Model file for the job. Use its own axes, mm. A direction names the side the tool comes from. Round coordinates to 2 decimals unless told otherwise and drop trailing zeros. Loops run counter-clockwise (first coordinate to the right, second up) from the corner with the lowest first, then second, coordinate; pieces in that order, holes last. Notation, with made-up numbers: (6, 0) - (42, 0) arc R33 cw to (42, 29) - close; hole circle Ø4 at (73, -22.5). An arc over 180 degrees is marked (long way). Answer as a JSON object with one key per item and string values.
from build123d import *

# Parameters (mm, degrees)
BOSS_EXTRUDE1_DEPTH     = 5
SKETCH4_W               = 80
SKETCH4_H               = 80
BOSS_EXTRUDE2_DEPTH     = 5
CUT_EXTRUDE4_DEPTH      = 5
CUT_EXTRUDE4_DEPTH_BACK = 5
SKETCH6_R               = 2.5
SKETCH7_R               = 1.25
CUT_EXTRUDE5_DEPTH      = 5
SKETCH8_R               = 5
CUT_EXTRUDE6_DEPTH      = 10
BOSS_EXTRUDE3_START     = -5
BOSS_EXTRUDE3_DEPTH     = 5
FILLET1_R               = 2
FILLET2_R               = 2


with BuildPart() as part:
    # Sketch3 → Boss-Extrude1 (new body)
    with BuildSketch(Plane(origin=(0, 0, 0), x_dir=(1, 0, 0), z_dir=(0, 1, 0))):
        with BuildLine():
            Line((-60, 40), (-40, 60))
            ThreePointArc((-40, 60), (0, 42.5), (40, 60))
            Line((40, 60), (60, 40))
            ThreePointArc((60, 40), (42.5, 0), (60, -40))
            Line((60, -40), (40, -60))
            ThreePointArc((40, -60), (0, -42.5), (-40, -60))
            Line((-40, -60), (-60, -40))
            ThreePointArc((-60, -40), (-42.5, 0), (-60, 40))
        make_face()
    extrude(amount=BOSS_EXTRUDE1_DEPTH)

    # Sketch4 → Boss-Extrude2 (add)
    with BuildSketch(Plane(origin=(0, 5, 0), x_dir=(1, 0, 0), z_dir=(0, 1, 0))):
        Rectangle(SKETCH4_W, SKETCH4_H)
    extrude(amount=BOSS_EXTRUDE2_DEPTH)

    # Sketch6 → Cut-Extrude4 (cut, two sides: drawn at the far end of the back side and taken through both)
    with BuildSketch(Plane(origin=(0, 5, 0), x_dir=(1, 0, 0), z_dir=(0, 1, 0)).offset(-CUT_EXTRUDE4_DEPTH_BACK)):
        with Locations(Location((-35, 35, 0), (0, 0, 270))):
            Circle(SKETCH6_R)
        with Locations(Location((35, 35, 0), (0, 0, 90))):
            Circle(SKETCH6_R)
        with Locations(Location((35, -35, 0), (0, 0, 270))):
            Circle(SKETCH6_R)
        with Locations(Location((-35, -35, 0), (0, 0, 90))):
            Circle(SKETCH6_R)
    extrude(amount=CUT_EXTRUDE4_DEPTH + CUT_EXTRUDE4_DEPTH_BACK, mode=Mode.SUBTRACT)

    # Sketch7 → Cut-Extrude5 (cut)
    with BuildSketch(Plane(origin=(0, 5, 0), x_dir=(1, 0, 0), z_dir=(0, 1, 0))):
        with BuildLine():
            Line((-47.878679656, 50.707106781), (-49.292893219, 49.292893219))
            Line((-49.292893219, 49.292893219), (-40.807611845, 40.807611845))
            Line((-40.807611845, 40.807611845), (-39.393398282, 42.221825407))
            ThreePointArc((-39.393398282, 42.221825407), (-39.100505063, 42.928932188), (-39.393398282, 43.636038969))
            Line((-39.393398282, 43.636038969), (-46.464466094, 50.707106781))
            ThreePointArc((-46.464466094, 50.707106781), (-47.171572875, 51), (-47.878679656, 50.707106781))
        make_face()
        with BuildLine():
            Line((-40.807611845, 40.807611845), (-49.292893219, 49.292893219))
            Line((-49.292893219, 49.292893219), (-50.707106781, 47.878679656))
            ThreePointArc((-50.707106781, 47.878679656), (-51, 47.171572875), (-50.707106781, 46.464466094))
            Line((-50.707106781, 46.464466094), (-43.636038969, 39.393398282))
            ThreePointArc((-43.636038969, 39.393398282), (-42.928932188, 39.100505063), (-42.221825407, 39.393398282))
            Line((-42.221825407, 39.393398282), (-40.807611845, 40.807611845))
        make_face()
        with Locations(Location((-53.181980515, 41.868272016, 0), (0, 0, 270))):
            Circle(SKETCH7_R)
        with Locations(Location((-48.232233047, 36.918524548, 0), (0, 0, 270))):
            Circle(SKETCH7_R)
        with Locations(Location((-41.868272016, 53.181980515, 0), (0, 0, 270))):
            Circle(SKETCH7_R)
        with Locations(Location((-36.918524548, 48.232233047, 0), (0, 0, 270))):
            Circle(SKETCH7_R)
        with BuildLine():
            Line((-39.393398282, -42.221825407), (-40.807611845, -40.807611845))
            Line((-40.807611845, -40.807611845), (-49.292893219, -49.292893219))
            Line((-49.292893219, -49.292893219), (-47.878679656, -50.707106781))
            ThreePointArc((-47.878679656, -50.707106781), (-47.171572875, -51), (-46.464466094, -50.707106781))
            Line((-46.464466094, -50.707106781), (-39.393398282, -43.636038969))
            ThreePointArc((-39.393398282, -43.636038969), (-39.100505063, -42.928932188), (-39.393398282, -42.221825407))
        make_face()
        with BuildLine():
            Line((-49.292893219, -49.292893219), (-40.807611845, -40.807611845))
            Line((-40.807611845, -40.807611845), (-42.221825407, -39.393398282))
            ThreePointArc((-42.221825407, -39.393398282), (-42.928932188, -39.100505063), (-43.636038969, -39.393398282))
            Line((-43.636038969, -39.393398282), (-50.707106781, -46.464466094))
            ThreePointArc((-50.707106781, -46.464466094), (-51, -47.171572875), (-50.707106781, -47.878679656))
            Line((-50.707106781, -47.878679656), (-49.292893219, -49.292893219))
        make_face()
        with Locations(Location((-53.181980515, -41.868272016, 0), (0, 0, 270))):
            Circle(SKETCH7_R)
        with Locations(Location((-48.232233047, -36.918524548, 0), (0, 0, 270))):
            Circle(SKETCH7_R)
        with Locations(Location((-41.868272016, -53.181980515, 0), (0, 0, 270))):
            Circle(SKETCH7_R)
        with BuildLine():
            Line((49.292893219, -49.292893219), (40.807611845, -40.807611845))
            Line((40.807611845, -40.807611845), (39.393398282, -42.221825407))
            ThreePointArc((39.393398282, -42.221825407), (39.100505063, -42.928932188), (39.393398282, -43.636038969))
            Line((39.393398282, -43.636038969), (46.464466094, -50.707106781))
            ThreePointArc((46.464466094, -50.707106781), (47.171572875, -51), (47.878679656, -50.707106781))
            Line((47.878679656, -50.707106781), (49.292893219, -49.292893219))
        make_face()
        with BuildLine():
            Line((42.221825407, -39.393398282), (40.807611845, -40.807611845))
            Line((40.807611845, -40.807611845), (49.292893219, -49.292893219))
            Line((49.292893219, -49.292893219), (50.707106781, -47.878679656))
            ThreePointArc((50.707106781, -47.878679656), (51, -47.171572875), (50.707106781, -46.464466094))
            Line((50.707106781, -46.464466094), (43.636038969, -39.393398282))
            ThreePointArc((43.636038969, -39.393398282), (42.928932188, -39.100505063), (42.221825407, -39.393398282))
        make_face()
        with Locations(Location((53.181980515, -41.868272016, 0), (0, 0, 270))):
            Circle(SKETCH7_R)
        with BuildLine():
            Line((39.393398282, 42.221825407), (40.807611845, 40.807611845))
            Line((40.807611845, 40.807611845), (49.292893219, 49.292893219))
            Line((49.292893219, 49.292893219), (47.878679656, 50.707106781))
            ThreePointArc((47.878679656, 50.707106781), (47.171572875, 51), (46.464466094, 50.707106781))
            Line((46.464466094, 50.707106781), (39.393398282, 43.636038969))
            ThreePointArc((39.393398282, 43.636038969), (39.100505063, 42.928932188), (39.393398282, 42.221825407))
        make_face()
        with BuildLine():
            Line((49.292893219, 49.292893219), (40.807611845, 40.807611845))
            Line((40.807611845, 40.807611845), (42.221825407, 39.393398282))
            ThreePointArc((42.221825407, 39.393398282), (42.928932188, 39.100505063), (43.636038969, 39.393398282))
            Line((43.636038969, 39.393398282), (50.707106781, 46.464466094))
            ThreePointArc((50.707106781, 46.464466094), (51, 47.171572875), (50.707106781, 47.878679656))
            Line((50.707106781, 47.878679656), (49.292893219, 49.292893219))
        make_face()
        with Locations(Location((41.868272016, 53.181980515, 0), (0, 0, 270))):
            Circle(SKETCH7_R)
        with Locations(Location((36.918524548, 48.232233047, 0), (0, 0, 270))):
            Circle(SKETCH7_R)
        with Locations(Location((53.181980515, 41.868272016, 0), (0, 0, 270))):
            Circle(SKETCH7_R)
        with Locations(Location((48.232233047, 36.918524548, 0), (0, 0, 270))):
            Circle(SKETCH7_R)
        with Locations(Location((-36.918524548, -48.232233047, 0), (0, 0, 90))):
            Circle(SKETCH7_R)
        with Locations(Location((48.232233047, -36.918524548, 0), (0, 0, 90))):
            Circle(SKETCH7_R)
        with Locations(Location((41.868272016, -53.181980515, 0), (0, 0, 270))):
            Circle(SKETCH7_R)
        with Locations(Location((36.918524548, -48.232233047, 0), (0, 0, 270))):
            Circle(SKETCH7_R)
    extrude(amount=-CUT_EXTRUDE5_DEPTH, mode=Mode.SUBTRACT)

    # Sketch8 → Cut-Extrude6 (cut)
    with BuildSketch(Plane(origin=(0, 0, 0), x_dir=(1, 0, 0), z_dir=(0, 1, 0))):
        with Locations(Location((0, 0, 0), (0, 0, 270))):
            Circle(SKETCH8_R)
    extrude(amount=CUT_EXTRUDE6_DEPTH, mode=Mode.SUBTRACT)

    # Sketch9 → Boss-Extrude3 (add)
    with BuildSketch(Plane(origin=(0, 5, 0), x_dir=(1, 0, 0), z_dir=(0, 1, 0)).offset(BOSS_EXTRUDE3_START)):
        with BuildLine():
            Line((-15, -96.964285714), (15, -96.964285714))
            add(Edge.make_bspline(
                [(15, -96.964285714), (15.040974101, -60.242963076), (40, -60)],
                knots=[0, 0, 0, 1, 1, 1], degree=2))
            ThreePointArc((40, -60), (0, -42.5), (-40, -60))
            add(Edge.make_bspline(
                [(-15, -96.964285714), (-15.040974101, -60.242963076), (-40, -60)],
                knots=[0, 0, 0, 1, 1, 1], degree=2))
        make_face()
    extrude(amount=BOSS_EXTRUDE3_DEPTH)

    # Fillet1
    fillet1_edges = [part.edges().sort_by_distance(p)[0] for p in [
        (-40, 2.5, 60),
        (-60, 2.5, 40),
        (-60, 2.5, -40),
        (-40, 2.5, -60),
        (40, 2.5, -60),
        (60, 2.5, -40),
        (-15, 2.5, 96.964285714),
        (60, 2.5, 40),
        (40, 2.5, 60),
        (15, 2.5, 96.964285714),
    ]]
    fillet(fillet1_edges, radius=FILLET1_R)

    # Fillet2
    fillet2_edges = [part.edges().sort_by_distance(p)[0] for p in [
        (40, 7.5, 40),
        (40, 7.5, -40),
        (-40, 7.5, -40),
        (-40, 7.5, 40),
    ]]
    fillet(fillet2_edges, radius=FILLET2_R)


solid = part.part
1) Probe probe 1 along Y at (x, z) = (-9, 89); probe 2 along Z at (x, y) = (-28, 8.75); probe 3 along X at (y, z) = (2, 8). List the from-to ranges inside material, lowest first.
Values follow:
{"probe 1": "0 to 5", "probe 2": "-40 to 40", "probe 3": "-43.09 to 43.09"}
2) Tool access for faces 4 (the flat face through (42.88, 2.54, 47.12)), 5 (the flat face through (-1, 7, 40)), 6 (the flat face through (-1, 7, -40)): list every direction of +Z, -Z, +X, -X, +Y, -Y with a clear straight run to the whole face (end or side of a thin tool).
Values follow:
{"face 4": "+Y, -Y", "face 5": "+Z, +X, -X, +Y", "face 6": "-Z, +X, -X, +Y"}
3) Slice it at A-A on z = 0. List the corners of the cut face in (x, y), then the cut area to 3 significant figures.
Values follow:
{"outline": "(-42.5, 0) - (-5, 0) - (-5, 10) - (-40, 10) - (-40, 5) - (-42.5, 5) - close; (5, 0) - (42.5, 0) - (42.5, 5) - (40, 5) - (40, 10) - (5, 10) - close", "area": "725 mm²"}
4) Slice it at B-B on y = 7. List the corners of the cut face in (x, z), then the cut area to 3 significant figures.
Values follow:
{"outline": "(-40, -38) arc R2 ccw to (-38, -40) - (38, -40) arc R2 ccw to (40, -38) - (40, 38) arc R2 ccw to (38, 40) - (-38, 40) arc R2 ccw to (-40, 38) - close; hole circle Ø5 at (-35, -35); hole circle Ø5 at (-35, 35); hole circle Ø10 at (0, 0); hole circle Ø5 at (35, -35); hole circle Ø5 at (35, 35)", "area": "6,240 mm²"}
5) Drop flat-ended pins along their axis: P1, Ø1.5, axis at x = -36.92, z = 48.23, coming from the +Y side; P2, Ø5, axis at y = 5, z = -8, coming from the +X side; P3, Ø2, axis at x = -24, y = 5.5, coming from the +Z side; P4, Ø2, axis at y = 2, z = 23.5, coming from the +X side. Give the stop position or say it passes through.
Values follow:
{"P1": "through", "P2": "x = 43.52", "P3": "z = 66.96", "P4": "x = 48.32"}
6) Two-plate mould, pull along X, no slides. Class faces 1 (the flat face through (-40, 7, 1)), 2 (the flat face through (40, 7, 1)), 3 (the cylindrical face through (34.249, 4.93, -37.385)): pulls with the +X half, pulls with the -X half, needs draft (parallel to the pull), parting line crosses it, or undercut.
Values follow:
{"face 1": "pulls with the -X half", "face 2": "pulls with the +X half", "face 3": "undercut"}
